from build123d import *

# Parameters (mm, degrees)
F0_R     = 1.778
F1_DEPTH = 2.54
F2_R     = 5.08
F3_R     = 1.016


with BuildPart() as f1:
    # F0 (on Front) → F1 (new body)
    with BuildSketch(Plane.XZ):
        with BuildLine():
            ThreePointArc((7.605604, -0.468175), (7.6164, -0.234198), (7.62, 0))
            ThreePointArc((7.62, 0), (7.6164, 0.234198), (7.605604, 0.468175))
            ThreePointArc((7.605604, 0.468175), (7.247051, 2.354709), (6.428249, 4.0917))
            ThreePointArc((6.428249, 4.0917), (6.164709, 4.478924), (5.877877, 4.849223))
            ThreePointArc((5.877877, 4.849223), (4.478924, 6.164709), (2.795522, 7.088685))
            ThreePointArc((2.795522, 7.088685), (2.354709, 7.247051), (1.905, 7.378033))
            ThreePointArc((1.905, 7.378033), (0, 7.62), (-1.905, 7.378033))
            ThreePointArc((-1.905, 7.378033), (-2.354709, 7.247051), (-2.795522, 7.088685))
            ThreePointArc((-2.795522, 7.088685), (-4.478924, 6.164709), (-5.877877, 4.849223))
            ThreePointArc((-5.877877, 4.849223), (-6.164709, 4.478924), (-6.428249, 4.0917))
            ThreePointArc((-6.428249, 4.0917), (-7.247051, 2.354709), (-7.605604, 0.468175))
            ThreePointArc((-7.605604, 0.468175), (-7.62, 0), (-7.605604, -0.468175))
            ThreePointArc((-7.605604, -0.468175), (-7.247051, -2.354709), (-6.428249, -4.0917))
            ThreePointArc((-6.428249, -4.0917), (-6.164709, -4.478924), (-5.877877, -4.849223))
            ThreePointArc((-5.877877, -4.849223), (-4.478924, -6.164709), (-2.795522, -7.088685))
            ThreePointArc((-2.795522, -7.088685), (-2.354709, -7.247051), (-1.905, -7.378033))
            ThreePointArc((-1.905, -7.378033), (0, -7.62), (1.905, -7.378033))
            ThreePointArc((1.905, -7.378033), (2.354709, -7.247051), (2.795522, -7.088685))
            ThreePointArc((2.795522, -7.088685), (4.478924, -6.164709), (5.877877, -4.849223))
            ThreePointArc((5.877877, -4.849223), (6.164709, -4.478924), (6.428249, -4.0917))
            ThreePointArc((6.428249, -4.0917), (7.247051, -2.354709), (7.605604, -0.468175))
        make_face()
        Circle(F0_R, mode=Mode.SUBTRACT)
        with BuildLine():
            ThreePointArc((6.428249, 4.0917), (7.247051, 2.354709), (7.605604, 0.468175))
            Line((7.605604, 0.468175), (9.689785, 1.412438))
            Line((9.689785, 1.412438), (11.830752, 3.04283))
            Line((11.830752, 3.04283), (11.35981, 4.49224))
            Line((11.35981, 4.49224), (8.66941, 4.552826))
            Line((8.66941, 4.552826), (6.428249, 4.0917))
        make_face()
        with BuildLine():
            Line((9.689785, -1.412438), (7.605604, -0.468175))
            ThreePointArc((7.605604, -0.468175), (7.247051, -2.354709), (6.428249, -4.0917))
            Line((6.428249, -4.0917), (8.66941, -4.552826))
            Line((8.66941, -4.552826), (11.35981, -4.49224))
            Line((11.35981, -4.49224), (11.830752, -3.04283))
            Line((11.830752, -3.04283), (9.689785, -1.412438))
        make_face()
        with BuildLine():
            ThreePointArc((2.795522, 7.088685), (4.478924, 6.164709), (5.877877, 4.849223))
            Line((5.877877, 4.849223), (7.00899, 6.838199))
            Line((7.00899, 6.838199), (7.782749, 9.415643))
            Line((7.782749, 9.415643), (6.549807, 10.311428))
            Line((6.549807, 10.311428), (4.337616, 8.779065))
            Line((4.337616, 8.779065), (2.795522, 7.088685))
        make_face()
        with BuildLine():
            Line((7.00899, -6.838199), (5.877877, -4.849223))
            ThreePointArc((5.877877, -4.849223), (4.478924, -6.164709), (2.795522, -7.088685))
            Line((2.795522, -7.088685), (4.337616, -8.779065))
            Line((4.337616, -8.779065), (6.549807, -10.311428))
            Line((6.549807, -10.311428), (7.782749, -9.415643))
            Line((7.782749, -9.415643), (7.00899, -6.838199))
        make_face()
        with BuildLine():
            ThreePointArc((-1.905, 7.378033), (0, 7.62), (1.905, 7.378033))
            Line((1.905, 7.378033), (1.651, 9.652))
            Line((1.651, 9.652), (0.762, 12.192))
            Line((0.762, 12.192), (-0.762, 12.192))
            Line((-0.762, 12.192), (-1.651, 9.652))
            Line((-1.651, 9.652), (-1.905, 7.378033))
        make_face()
        with BuildLine():
            Line((1.651, -9.652), (1.905, -7.378033))
            ThreePointArc((1.905, -7.378033), (0, -7.62), (-1.905, -7.378033))
            Line((-1.905, -7.378033), (-1.651, -9.652))
            Line((-1.651, -9.652), (-0.762, -12.192))
            Line((-0.762, -12.192), (0.762, -12.192))
            Line((0.762, -12.192), (1.651, -9.652))
        make_face()
        with BuildLine():
            ThreePointArc((-5.877877, 4.849223), (-4.478924, 6.164709), (-2.795522, 7.088685))
            Line((-2.795522, 7.088685), (-4.337616, 8.779065))
            Line((-4.337616, 8.779065), (-6.549807, 10.311428))
            Line((-6.549807, 10.311428), (-7.782749, 9.415643))
            Line((-7.782749, 9.415643), (-7.00899, 6.838199))
            Line((-7.00899, 6.838199), (-5.877877, 4.849223))
        make_face()
        with BuildLine():
            Line((-4.337616, -8.779065), (-2.795522, -7.088685))
            ThreePointArc((-2.795522, -7.088685), (-4.478924, -6.164709), (-5.877877, -4.849223))
            Line((-5.877877, -4.849223), (-7.00899, -6.838199))
            Line((-7.00899, -6.838199), (-7.782749, -9.415643))
            Line((-7.782749, -9.415643), (-6.549807, -10.311428))
            Line((-6.549807, -10.311428), (-4.337616, -8.779065))
        make_face()
        with BuildLine():
            ThreePointArc((-7.605604, 0.468175), (-7.247051, 2.354709), (-6.428249, 4.0917))
            Line((-6.428249, 4.0917), (-8.66941, 4.552826))
            Line((-8.66941, 4.552826), (-11.35981, 4.49224))
            Line((-11.35981, 4.49224), (-11.830752, 3.04283))
            Line((-11.830752, 3.04283), (-9.689785, 1.412438))
            Line((-9.689785, 1.412438), (-7.605604, 0.468175))
        make_face()
        with BuildLine():
            Line((-8.66941, -4.552826), (-6.428249, -4.0917))
            ThreePointArc((-6.428249, -4.0917), (-7.247051, -2.354709), (-7.605604, -0.468175))
            Line((-7.605604, -0.468175), (-9.689785, -1.412438))
            Line((-9.689785, -1.412438), (-11.830752, -3.04283))
            Line((-11.830752, -3.04283), (-11.35981, -4.49224))
            Line((-11.35981, -4.49224), (-8.66941, -4.552826))
        make_face()
    extrude(amount=F1_DEPTH)

    # F2
    f2_edges = [f1.edges().sort_by_distance(p)[0] for p in [
        (7.00899, -1.27, 6.838199),
        (4.337616, -1.27, 8.779065),
        (1.651, -1.27, 9.652),
        (-4.337616, -1.27, 8.779065),
        (-8.66941, -1.27, 4.552826),
        (-9.689785, -1.27, -1.412438),
        (-7.00899, -1.27, -6.838199),
        (-1.651, -1.27, -9.652),
        (4.337616, -1.27, -8.779065),
        (8.66941, -1.27, -4.552826),
        (9.689785, -1.27, 1.412438),
        (9.689785, -1.27, -1.412438),
        (8.66941, -1.27, 4.552826),
        (-1.651, -1.27, 9.652),
        (-7.00899, -1.27, 6.838199),
        (-9.689785, -1.27, 1.412438),
        (-8.66941, -1.27, -4.552826),
        (-4.337616, -1.27, -8.779065),
        (1.651, -1.27, -9.652),
        (7.00899, -1.27, -6.838199),
    ]]
    fillet(f2_edges, radius=F2_R)

    # F3
    f3_edges = [f1.edges().sort_by_distance(p)[0] for p in [
        (0.762, -1.27, 12.192),
        (-0.762, -1.27, 12.192),
        (-6.549807, -1.27, 10.311428),
        (-7.782749, -1.27, 9.415643),
        (-11.35981, -1.27, 4.49224),
        (6.549807, -1.27, 10.311428),
        (7.782749, -1.27, 9.415643),
        (11.35981, -1.27, 4.49224),
        (-11.830752, -1.27, 3.04283),
        (-11.830752, -1.27, -3.04283),
        (-11.35981, -1.27, -4.49224),
        (-7.782749, -1.27, -9.415643),
        (-6.549807, -1.27, -10.311428),
        (-0.762, -1.27, -12.192),
        (0.762, -1.27, -12.192),
        (6.549807, -1.27, -10.311428),
        (7.782749, -1.27, -9.415643),
        (11.830752, -1.27, -3.04283),
        (11.35981, -1.27, -4.49224),
        (11.830752, -1.27, 3.04283),
    ]]
    fillet(f3_edges, radius=F3_R)


solid = f1.part
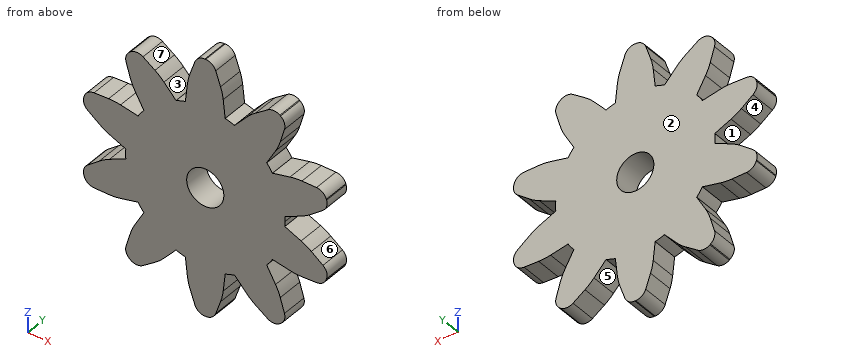
Design review of the part built by this model. Coordinates are the model's own, in mm. Face numbers are marked on the shaded views. A direction names the side the tool comes from. Give positions to 0.01 mm unless a question says otherwise; leave off trailing zeros. Loops run counter-clockwise (first coordinate to the right, second up) from the corner with the lowest first, then second, coordinate; pieces in that order, holes last. Notation, with made-up numbers: (38, 86) -> (89, 86) arc R30 cw to (89, 112) -> close; hole circle Ø8 at (-34.75, 54). An arc over 180 degrees is marked (long way). One line per question, with ' | ' between items. Start each with the question number.
(1) We need section B-B (z = -10.5). State the section outline as (x, y) points.
(2) Insertion check: P1, Ø1.5, axis at x = 6.5, y = -2, coming from the +Z side. The pin has a flat end and moves straight along its axis. Give the tip position at first contact, or say it passes through.
(3) For the marked faces 4, 5, 6 and 7, list the 3-axis set-ups (+Z, -Z, +X, -X, +Y, -Y) from which the entire face can be reached by the end or side of a thin tool; tool diameter is ignored.
(4) Draft analysis for pull direction Z (two halves, no side actions). For the marked faces 1, 2 and 3, state which applies: +Z half, -Z half, draft (parallel to the pull), parting line (faces both ways), or undercut.
(5) For line 1 (Z direction, x = 0, y = -1.15); line 2 (X direction, y = -1.7, z = 8); line 3 (X direction, y = -1.4, z = 8.5), list the stretches that pass through material, from the lowest coordinate up.
(6) We need section A-A (x = -8.75). State the section outline as (y, z) points.
(7) We need section C-C (x = -3.25). State the section outline as (y, z) points, and give its area (3 significant figures).
The answers:
1) outline: (-1.35, -2.54) -> (1.35, -2.54) -> (1.35, 0) -> (-1.35, 0) -> close
2) P1: stops at z = 10.08
3) face 4: -X, +Y, -Y | face 5: -Z, +Y, -Y | face 6: +X, +Y, -Y | face 7: +Z, +Y, -Y
4) face 1: undercut | face 2: draft | face 3: +Z half
5) line 1: z = -12.19 to -1.78, 1.78 to 12.19 | line 2: x = -7.36 to -3.63, -1.84 to 1.84, 3.63 to 7.36 | line 3: x = -7.51 to -4.09, -1.78 to 1.78, 4.09 to 7.51
6) outline: (-2.54, -4.53) -> (0, -4.53) -> (0, -0.99) -> (-2.54, -0.99) -> close; (-2.54, 0.99) -> (0, 0.99) -> (0, 4.53) -> (-2.54, 4.53) -> close
7) outline: (-2.54, -7.59) -> (0, -7.59) -> (0, 7.59) -> (-2.54, 7.59) -> close | area: 38.5 mm^2
